The listing builds one solid part. Answer for the finished solid, in the listing's coordinates (mm). Face numbers are marked on the shaded views. A direction names the side the tool comes from. Round coordinates to 2 decimals unless told otherwise and drop trailing zeros. Loops run counter-clockwise (first coordinate to the right, second up) from the corner with the lowest first, then second, coordinate; pieces in that order, holes last. Notation, with made-up numbers: (-35, 51) - (7, 51) arc R18 cw to (7, 75) - close; hole circle Ø3 at (89, 27.25). An arc over 180 degrees is marked (long way). One line per item, written item: value.
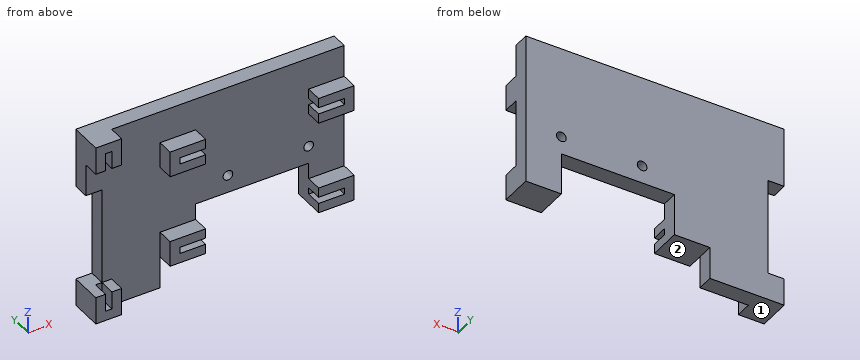
```python
from build123d import *

# Parameters (mm, degrees)
SKETCH1_W               = 8
SKETCH1_H               = 57
SKETCH1_W_2             = 2
SKETCH1_H_2             = 51
BOSS_EXTRUDE1_DEPTH     = 5
SKETCH2_W               = 80
SKETCH2_H               = 57
BOSS_EXTRUDE2_DEPTH     = 5
SKETCH3_W               = 40
SKETCH3_H               = 10
CUT_EXTRUDE1_DEPTH      = 8
SKETCH4_W               = 57
SKETCH4_H               = 8
SKETCH4_W_2             = 51
SKETCH4_H_2             = 2
BOSS_EXTRUDE3_DEPTH     = 5
SKETCH5_W               = 35
SKETCH5_H               = 10
CUT_EXTRUDE2_DEPTH      = 8
SKETCH6_W               = 35
SKETCH6_H               = 5
CUT_EXTRUDE3_DEPTH      = 6
CUT_EXTRUDE3_DEPTH_BACK = 6
SKETCH7_W               = 30
SKETCH7_H               = 5
CUT_EXTRUDE5_DEPTH      = 5
SKETCH8_R               = 1.5
CUT_EXTRUDE6_DEPTH      = 1
CUT_EXTRUDE6_DEPTH_BACK = 11


with BuildPart() as part:
    # Sketch1 → Boss-Extrude1 (new body)
    with BuildSketch(Plane(origin=(0, 0, 0), x_dir=(1, 0, 0), z_dir=(0, 1, 0))):
        Rectangle(SKETCH1_W, SKETCH1_H)
        Rectangle(SKETCH1_W_2, SKETCH1_H_2, mode=Mode.SUBTRACT)
    extrude(amount=BOSS_EXTRUDE1_DEPTH)

    # Sketch2 → Boss-Extrude2 (add)
    with BuildSketch(Plane(origin=(0, 5, 0), x_dir=(1, 0, 0), z_dir=(0, 1, 0))):
        with Locations((36, 0)):
            Rectangle(SKETCH2_W, SKETCH2_H)
    extrude(amount=BOSS_EXTRUDE2_DEPTH)

    # Sketch3 → Cut-Extrude1 (cut)
    with BuildSketch(Plane.ZY.offset(4)):
        Rectangle(SKETCH3_W, SKETCH3_H)
    extrude(amount=-CUT_EXTRUDE1_DEPTH, mode=Mode.SUBTRACT)

    # Sketch4 → Boss-Extrude3 (add)
    with BuildSketch(Plane.XZ.offset(-5)):
        with Locations((47.5, 14.5)):
            Rectangle(SKETCH4_W, SKETCH4_H)
        with Locations((47.5, 14.5)):
            Rectangle(SKETCH4_W_2, SKETCH4_H_2, mode=Mode.SUBTRACT)
    boss_extrude3 = extrude(amount=BOSS_EXTRUDE3_DEPTH)

    # Sketch5 → Cut-Extrude2 (cut)
    with BuildSketch(Plane.XY.offset(18.5)):
        with Locations((47.5, 0)):
            Rectangle(SKETCH5_W, SKETCH5_H)
    cut_extrude2 = extrude(amount=-CUT_EXTRUDE2_DEPTH, mode=Mode.SUBTRACT)

    # Mirror2: Boss-Extrude3, Cut-Extrude2 across plane
    add(boss_extrude3.mirror(Plane.XY))
    add(cut_extrude2.mirror(Plane.XY), mode=Mode.SUBTRACT)

    # Sketch6 → Cut-Extrude3 (cut, two sides)
    with BuildSketch(Plane.XZ.offset(-5)) as cut_extrude3_sk:
        Polygon((30, -18.5), (65, -18.5), (65, -15.5), (65, -13.5), (65, -10.5), (30, -10.5), (30, -13.5), (30, -15.5), align=None)
        Polygon((19, -28.5), (76, -28.5), (76, -18.5), (65, -18.5), (30, -18.5), (19, -18.5), align=None)
        with Locations((47.5, -8)):
            Rectangle(SKETCH6_W, SKETCH6_H)
    extrude(amount=CUT_EXTRUDE3_DEPTH, mode=Mode.SUBTRACT)
    extrude(cut_extrude3_sk.sketch, amount=-CUT_EXTRUDE3_DEPTH_BACK, mode=Mode.SUBTRACT)

    # Sketch7 → Cut-Extrude5 (cut)
    with BuildSketch(Plane.ZY.offset(4)):
        with Locations((-5, 7.5)):
            Rectangle(SKETCH7_W, SKETCH7_H)
    extrude(amount=-CUT_EXTRUDE5_DEPTH, mode=Mode.SUBTRACT)

    # Sketch8 → Cut-Extrude6 (cut, two sides)
    with BuildSketch(Plane(origin=(0, 10, 0), x_dir=(1, 0, 0), z_dir=(0, 1, 0))) as cut_extrude6_sk:
        with Locations((65, 0)):
            Circle(SKETCH8_R)
        with Locations((40, 0)):
            Circle(SKETCH8_R)
    extrude(amount=CUT_EXTRUDE6_DEPTH, mode=Mode.SUBTRACT)
    extrude(cut_extrude6_sk.sketch, amount=-CUT_EXTRUDE6_DEPTH_BACK, mode=Mode.SUBTRACT)


solid = part.part
```
1) A cutting plane is placed at B-B on x = 40. Give the vertices of the cut face in (y, z), and give its area (3 significant figures).
Final values:
outline: (5, -5.5) - (10, -5.5) - (10, -1.5) - (5, -1.5) - close; (5, 1.5) - (10, 1.5) - (10, 28.5) - (5, 28.5) - close
area: 155 mm2
2) Each of these flat-tipped pins is pushed along its axis until it touches: pin 1 Ø1 at (y, z) = (3, 7) entering from -X; pin 2 Ø1.5 at (x, z) = (56, 3) entering from -Y; pin 3 Ø3.5 at (y, z) = (3, 11.5) entering from -X; pin 4 Ø2.5 at (x, y) = (27.5, 1.5) entering from -Z. Where does it stop, or does it pass through?
Final values:
pin 1: through
pin 2: y = 5
pin 3: x = 19
pin 4: z = -18.5
3) A cutting plane is placed at A-A on z = 0. Give the vertices of the cut face in (x, y), and give its area (3 significant figures).
Final values:
outline: (1, 5) - (38.5, 5) - (38.5, 10) - (1, 10) - close; (41.5, 5) - (63.5, 5) - (63.5, 10) - (41.5, 10) - close; (66.5, 5) - (76, 5) - (76, 10) - (66.5, 10) - close
area: 345 mm2
4) Consider L1, parallel to X at y = 7.3, z = 0; L2, parallel to Z at x = 40, y = 6.35; L3, parallel to X at y = 4, z = 16. Determine where each line is inside the solid, lowest interval first.
Final values:
L1: 1 to 38.5, 41.5 to 63.5, 66.5 to 76
L2: -5.5 to -1.5, 1.5 to 28.5
L3: 19 to 30, 65 to 76
5) For the marked faces 1 and 2, determine the directions among +Z, -Z, +X, -X, +Y, -Y from which every point of the face is accessible in a straight line to the end or side of a thin tool.
Final values:
face 1: -Z, +X, -X, +Y, -Y
face 2: -Z, +X, +Y, -Y
6) A cutting plane is placed at D-D on z = -14.5. Give the vertices of the cut face in (x, y).
Final values:
outline: (1, 5) - (19, 5) - (19, 0) - (22, 0) - (22, 5) - (30, 5) - (30, 10) - (1, 10) - close; (65, 5) - (73, 5) - (73, 0) - (76, 0) - (76, 10) - (65, 10) - close
7) A cutting plane is placed at C-C on y = 7.5. Give the vertices of the cut face in (x, z).
Final values:
outline: (-4, -28.5) - (19, -28.5) - (19, -18.5) - (30, -18.5) - (30, -5.5) - (65, -5.5) - (65, -18.5) - (76, -18.5) - (76, 28.5) - (-4, 28.5) - (-4, 10) - (1, 10) - (1, -20) - (-4, -20) - close; hole circle Ø3 at (40, 0); hole circle Ø3 at (65, 0)
